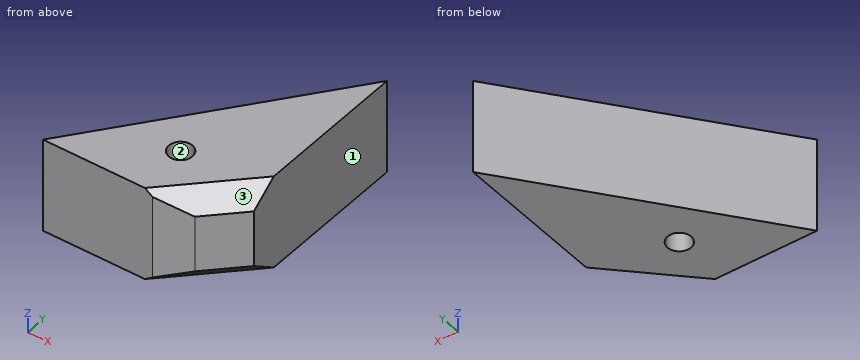
from build123d import *

# Parameters (mm, degrees)
F1_DEPTH = 25.4
F2_SIZE  = 12.7
F3_SIZE  = 5.08
F4_SIZE  = 5.08
F5_SIZE  = 5.08
F7_D     = 6.35


with BuildPart() as f1:
    # F0 (on Top) → F1 (new body)
    with BuildSketch(Plane.XY):
        Polygon((47.389537096, 60.6057569385), (0, 0), (47.389537096, 0), align=None)
    extrude(amount=F1_DEPTH)

    # F2
    f2_edges = [f1.edges().sort_by_distance(p)[0] for p in [
        (47.389537, 0, 12.7),
    ]]
    chamfer(f2_edges, length=F2_SIZE)

    # F3
    f3_edges = [f1.edges().sort_by_distance(p)[0] for p in [
        (41.039537, 6.35, 25.4),
    ]]
    chamfer(f3_edges, length=F3_SIZE)

    # F4
    f4_edges = [f1.edges().sort_by_distance(p)[0] for p in [
        (41.039537, 6.35, 0),
    ]]
    chamfer(f4_edges, length=F4_SIZE)

    # F5
    f5_edges = [f1.edges().sort_by_distance(p)[0] for p in [
        (34.689537, 0, 12.7),
    ]]
    chamfer(f5_edges, length=F5_SIZE)

    # F7 (through all)
    with Locations(Plane.XY.offset(25.4)):
        with Locations((26.0983891785, 14.7461835295)):
            Hole(F7_D / 2)


solid = f1.part
Verification items for the finished model (mm, model axes). Face numbers are marked on the shaded views. Coordinates: 2 decimals unless noted, no trailing zeros. Order: outer loops, then holes, each group sorted by start corner. A loop starts at its lowest first (then second) coordinate and runs counter-clockwise, first axis right, second up. Notation, with made-up numbers: M 23.5,23 L 30.5,23 A19 cw 30.5,47 Z; hole C 55.5,89 d9. An arc over 180 degrees is marked long. Write each question's results on one line, items separated by ' | '.
1) Section check A-A on z = 19.5. Record the cut outline in (x, y) (3 decimals).
Solved:
outline: M 0,0 L 29.61,0 L 38.282,3.592 L 47.39,12.7 L 47.39,60.606 Z; hole C 26.098,14.746 d6.35
2) Scan lines: line 1 along Y through (x, z) = (24.5, 24); line 2 along Y through (x, z) = (29, 8.5); line 3 along Y through (x, z) = (40, 2). Record each from-to range of solid material in increasing order. Write a range as [from, to].
Solved:
line 1: y = [0, 12], [17.49, 31.33] | line 2: y = [0, 13.46], [16.04, 37.09] | line 3: y = [9.67, 51.16]
3) Gauge pin test, flat ends, axial feed: pin 1 Ø1.5 at (y, z) = (40.5, 20.5) entering from -X; pin 2 Ø3 at (x, z) = (27, 8) entering from +Y; pin 3 Ø6 at (y, z) = (33, 14.5) entering from -X. Record the tip position at first contact, or that the pin passes through.
Solved:
pin 1: stops at x = 31.08 | pin 2: stops at y = 36.45 | pin 3: stops at x = 23.46
4) Section check D-D on x = 40.5. Record the cut outline in (y, z), plus the area to 3 significant figures.
Solved:
outline: M 5.81,5.08 L 12.99,0 L 51.79,0 L 51.79,25.4 L 12.99,25.4 L 5.81,20.32 Z | area: 1,130 mm²
5) Release check for a two-part mould opening along Y. For the marked faces 1, 2 and 3 record: pulls with the +Y half, pulls with the -Y half, needs draft (parallel to the pull), parting line crosses it, or undercut.
Solved:
face 1: needs draft | face 2: undercut | face 3: pulls with the -Y half
6) Section check B-B on x = 16. Record the cut outline in (y, z), plus the area to 3 significant figures.
Solved:
outline: M 0,0 L 20.46,0 L 20.46,25.4 L 0,25.4 Z | area: 520 mm²
7) Section check C-C on y = 49. Record the cut outline in (x, z).
Solved:
outline: M 38.31,0 L 47.39,0 L 47.39,25.4 L 38.31,25.4 Z
